Can you work these out from the drawing? Everything is in mm from the part's minimum corner. A direction names the side the tool comes from. Coordinates: 2 decimals unless noted, no trailing zeros. Loops run counter-clockwise (first coordinate to the right, second up) from the corner with the lowest first, then second, coordinate; pieces in that order, holes last.
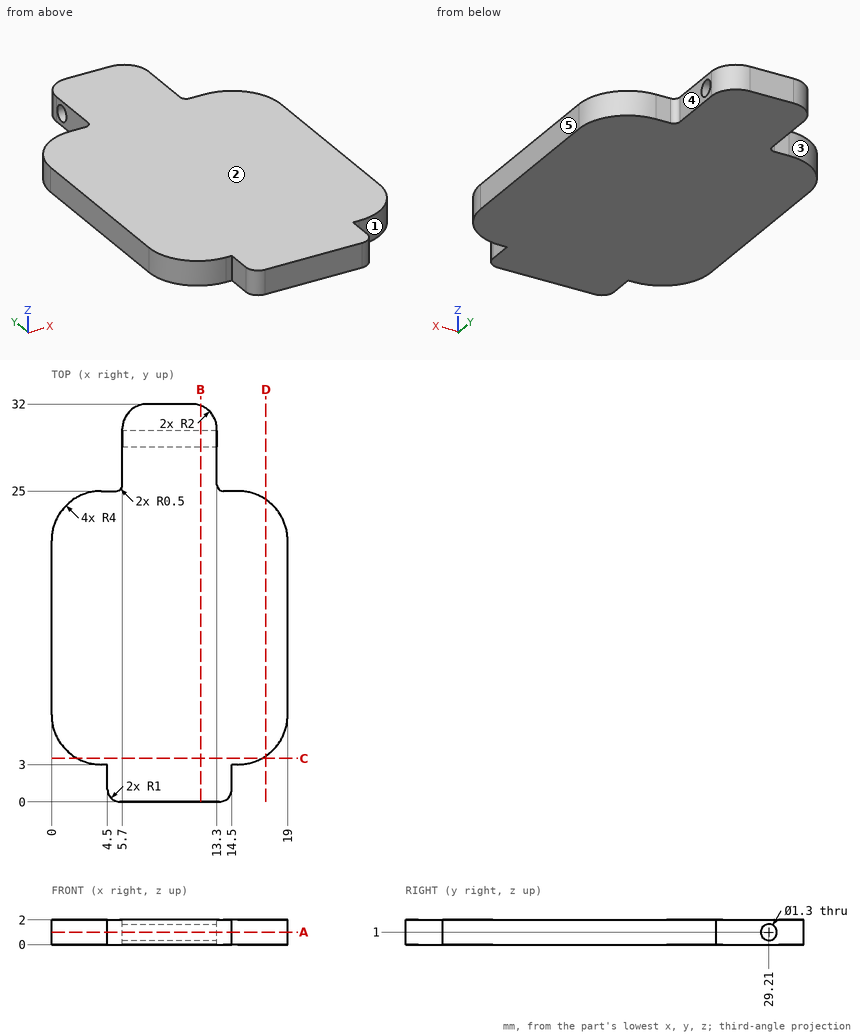
(1) Which directions (+Z, -Z, +X, -X, +Y, -Y) give clear straight access to the entire face, cutting with the end or side of a thin tool? Please do the marked faces 4 and 5.
Answers:
face 4: +Z, -Z, +X, +Y
face 5: +Z, -Z, +X, +Y, -Y
(2) Imagine slicing it at B-B, the plane x = 12. Write out the boundary of the cut face in (y, z).
Answers:
outline: (0, 0) - (31.87, 0) - (31.87, 2) - (0, 2) - close; hole circle Ø1.3 at (29.21, 1)
(3) Imagine slicing it at D-D, the plane x = 17.25. Write out the boundary of the cut face in (y, z), and give its area (3 significant figures).
Answers:
outline: (3.69, 0) - (24.31, 0) - (24.31, 2) - (3.69, 2) - close
area: 41.2 mm2
(4) I need wall thicknesses on probe 1 along Y at (x, z) = (3.75, 1.7); probe 2 along X at (y, z) = (27, 0.7); probe 3 along Y at (x, z) = (8.5, 0.85). Which ranges of each line are inside material? Lowest first, please.
Answers:
probe 1: y = 3.01 to 24.99
probe 2: x = 5.7 to 13.3
probe 3: y = 0 to 28.58, 29.84 to 32
(5) We'd pull the mould along Y, two halves only. Please class the marked faces 1, 2 and 3: +Y half, -Y half, draft (parallel to the pull), parting line (faces both ways), or undercut.
Answers:
face 1: -Y half
face 2: draft
face 3: +Y half
(6) For pin 1 (0.6 mm diameter, centred on y = 2.5, z = 1.5, fed in from -X); pin 2 (1 mm diameter, centred on y = 27, z = 1, fed in from +X), each with a flat end and sliding along its axis, tell me the tip position at first contact or that it passes through.
Answers:
pin 1: stops at x = 4.5
pin 2: stops at x = 13.3
(7) Imagine slicing it at C-C, the plane y = 3.5. Write out the boundary of the cut face in (x, z).
Answers:
outline: (2.06, 0) - (16.94, 0) - (16.94, 2) - (2.06, 2) - close
(8) Imagine slicing it at A-A, the plane z = 1. Write out the boundary of the cut face in (x, y).
Answers:
outline: (0, 7) arc R4 ccw to (4, 3) - (4.5, 3) - (4.5, 1) arc R1 ccw to (5.5, 0) - (13.5, 0) arc R1 ccw to (14.5, 1) - (14.5, 3) - (15, 3) arc R4 ccw to (19, 7) - (19, 21) arc R4 ccw to (15, 25) - (13.8, 25) arc R0.5 cw to (13.3, 25.5) - (13.3, 28.56) - (5.7, 28.56) - (5.7, 25.5) arc R0.5 cw to (5.2, 25) - (4, 25) arc R4 ccw to (0, 21) - close; (5.7, 29.86) - (13.3, 29.86) - (13.3, 30) arc R2 ccw to (11.3, 32) - (7.7, 32) arc R2 ccw to (5.7, 30) - close
